Here's how the part is built. I have some questions about the finished solid (model axes, mm). A direction names the side the tool comes from. Round coordinates to 2 decimals unless told otherwise and drop trailing zeros. Order: outer loops, then holes, each group sorted by start corner. A loop starts at its lowest first (then second) coordinate and runs counter-clockwise, first axis right, second up.
Autodesk Inventor part; units mm, degrees
ref_plane "YZ Plane" through (0, 0, 0) normal (1, 0, 0) x (0, 1, 0)
ref_plane "XZ Plane" through (0, 0, 0) normal (0, 1, 0) x (-1, 0, 0)
ref_plane "XY Plane" through (0, 0, 0) normal (0, 0, 1) x (1, 0, 0)
ref_plane "Arbeitsebene1" through (796.2209, 70.6141, -996.2958) normal (0, 0, -1) x (-1, 0, 0)
sketch "Skizze1" plane through (796.2209, 70.6141, -996.2958) normal (0, 0, -1) x (-1, 0, 0)
  line L0 (-3.9996, -76.75) -> (4.0004, -76.75) construction
  line L1 (-3.9996, 76.75) -> (-3.9996, -76.75) construction
  line L2 (4.0004, 76.75) -> (-3.9996, 76.75) construction
  line L3 (4.0004, 84.25) -> (4.0004, 76.75) construction
  line L4 (-37.8996, 84.25) -> (4.0004, 84.25) construction
  line L5 (-37.8996, 1.75) -> (-37.8996, 84.25) construction
  line L6 (-133.3996, 1.75) -> (-37.8996, 1.75) construction
  line L7 (-133.3996, -84.25) -> (-133.3996, 1.75) construction
  line L8 (4.0004, -84.25) -> (-133.3996, -84.25) construction
  line L9 (4.0004, -76.75) -> (4.0004, -84.25) construction
  line L10 (150.8004, -76.75) -> (142.8004, -76.75) construction
  line L11 (142.8004, -76.75) -> (142.8004, -84.25) construction
  line L12 (142.8004, -84.25) -> (280.2004, -84.25) construction
  line L13 (280.2004, -84.25) -> (280.2004, 1.75) construction
  line L14 (280.2004, 1.75) -> (184.7004, 1.75) construction
  line L15 (184.7004, 1.75) -> (184.7004, 84.25) construction
  line L16 (184.7004, 84.25) -> (142.8004, 84.25) construction
  line L17 (142.8004, 84.25) -> (142.8004, 76.75) construction
  line L18 (142.8004, 76.75) -> (150.8004, 76.75) construction
  line L19 (150.8004, 76.75) -> (150.8004, -76.75) construction
  line L20 (-5.9996, 76.75) -> (-5.9996, -76.75) construction
  line L21 (152.8004, 76.75) -> (152.8004, -76.75) construction
  line L22 (-5.9996, 76.75) -> (152.8004, 76.75) construction
  line L23 (-5.9996, -76.75) -> (152.8004, -76.75) construction
  line L24 (73.4004, -76.75) -> (73.4004, 76.75) construction
  line L25 (-5.8996, -76.65) -> (152.7004, -76.65)
  line L26 (152.7004, -76.65) -> (152.7004, 76.65)
  line L27 (152.7004, 76.65) -> (-5.8996, 76.65)
  line L28 (-5.8996, 76.65) -> (-5.8996, -76.65)
  line L29 (-5.8996, -76.65) -> (152.7004, 76.65) construction
  line L30 (152.7004, -76.65) -> (-5.8996, 76.65) construction
  point P0 (796.2209, -70.6141)
  point P1 (73.4004, 0)
  dimension "d24" = 0.1
  dimension "d25" = 0.1
extrude "Extrusion1" add sketch "Skizze1" along normal blind 2
sketch "Skizze2" plane through (796.2209, 70.6141, -996.2958) normal (0, 0, 1) x (1, 0, 0)
  line L0 (-152.8004, -76.75) -> (-142.8004, -76.75) construction
  line L1 (-142.8004, -66.75) -> (-152.8004, -66.75) construction
  line L2 (-142.8004, -76.75) -> (-142.8004, -66.75) construction
  line L3 (-152.8004, -66.75) -> (-152.8004, -76.75) construction
  line L4 (-4.0004, -66.75) -> (5.9996, -66.75) construction
  line L5 (-4.0004, -76.75) -> (-4.0004, -66.75) construction
  line L6 (5.9996, -66.75) -> (5.9996, -76.75) construction
  line L7 (5.9996, -76.75) -> (-4.0004, -76.75) construction
  line L8 (-152.8004, 66.75) -> (-142.8004, 66.75) construction
  line L9 (-142.8004, 66.75) -> (-142.8004, 76.75) construction
  line L10 (-142.8004, 76.75) -> (-152.8004, 76.75) construction
  line L11 (-152.8004, 76.75) -> (-152.8004, 66.75) construction
  line L12 (-4.0004, 66.75) -> (-4.0004, 76.75) construction
  line L13 (5.9996, 66.75) -> (-4.0004, 66.75) construction
  line L14 (-4.0004, 76.75) -> (5.9996, 76.75) construction
  line L15 (5.9996, 76.75) -> (5.9996, 66.75) construction
  line L16 (-142.9004, -76.65) -> (-152.7004, -76.65)
  line L17 (-152.7004, -76.65) -> (-152.7004, -66.85)
  line L18 (-152.7004, -66.85) -> (-142.9004, -66.85)
  line L19 (-142.9004, -66.85) -> (-142.9004, -76.65)
  line L20 (5.8996, -76.65) -> (-152.7004, -76.65)
  line L21 (5.8996, -76.65) -> (5.8996, -66.85)
  line L22 (5.8996, -66.85) -> (-3.9004, -66.85)
  line L23 (-3.9004, -66.85) -> (-3.9004, -76.65)
  line L24 (-3.9004, -76.65) -> (5.8996, -76.65)
  line L25 (5.8996, 76.65) -> (5.8996, -76.65)
  line L26 (-3.9004, 66.85) -> (-3.9004, 76.65)
  line L27 (-3.9004, 76.65) -> (5.8996, 76.65)
  line L28 (5.8996, 76.65) -> (5.8996, 66.85)
  line L29 (5.8996, 66.85) -> (-3.9004, 66.85)
  line L30 (-142.9004, 76.65) -> (-142.9004, 66.85)
  line L31 (-142.9004, 66.85) -> (-152.7004, 66.85)
  line L32 (-152.7004, 66.85) -> (-152.7004, 76.65)
  line L33 (-152.7004, 76.65) -> (-142.9004, 76.65)
  line L34 (-152.7004, 76.65) -> (5.8996, 76.65)
  point P0 (-796.2209, -70.6141)
extrude "Extrusion2" add sketch "Skizze2" along normal blind 3.5
sketch "Skizze3" plane through (796.2209, 70.6141, -992.7958) normal (0, 0, 1) x (1, 0, 0)
  circle A0 centre (0.9996, 71.75) radius 1.75 construction
  circle A1 centre (0.9996, -71.75) radius 1.75 construction
  circle A2 centre (-147.8004, 71.75) radius 1.75 construction
  circle A3 centre (-147.8004, -71.75) radius 1.75 construction
  line L0 (-142.9004, 66.85) -> (-142.9004, 76.65)
  line L1 (-142.9004, 76.65) -> (-152.7004, 76.65)
  line L2 (-152.7004, 76.65) -> (-152.7004, 66.85)
  line L3 (-152.7004, 66.85) -> (-142.9004, 66.85)
  circle A4 centre (-147.8004, 71.75) radius 1.5
  circle A5 centre (1.0996, 71.75) radius 1.5
  circle A6 centre (1.0996, -71.75) radius 1.5
  circle A7 centre (-147.8004, -71.75) radius 1.5
  point P0 (-796.2209, -70.6141)
extrude "Extrusion3" cut sketch "Skizze3" against normal blind 15.5 contours A4 | A5 | A6 | A7
sketch "Skizze4" plane through (796.2209, 70.6141, -998.2958) normal (0, 0, -1) x (-1, 0, 0)
  circle A0 centre (147.8004, 71.75) radius 1.5 construction
  circle A1 centre (147.8004, -71.75) radius 1.5 construction
  circle A2 centre (-1.0996, -71.75) radius 1.5 construction
  circle A3 centre (147.8004, -71.75) radius 2.85
  circle A4 centre (-1.0996, -71.75) radius 2.85
  circle A5 centre (147.8004, 71.75) radius 2.85
  circle A6 centre (-1.0996, 71.75) radius 2.85
  circle A7 centre (-1.0996, 71.75) radius 1.5 construction
  point P0 (796.2209, -70.6141)
  dimension "d27" = 5.7
  dimension "d28" = 5.7
  dimension "d29" = 5.7
  dimension "d30" = 5.7
extrude "Extrusion4" cut sketch "Skizze4" against normal blind 3.1
equation "\"d28\" = d27"
equation "\"d29\" = d27"
equation "\"d30\" = d27"
properties part number "Backplate-housing"
1. If we section it at A-A, the plane y = 130.5: Write out the boundary of the cut face in (x, z), and give its area (3 significant figures).
Evaluation:
outline: (643.52, -998.3) - (802.12, -998.3) - (802.12, -996.3) - (643.52, -996.3) - close
area: 317 mm2
2. If we mould it in two halves opening along Y, with no side actions, what happens to faces 1 (the flat face through (647, -2, -995.196)), 2 (the flat face through (792.32, -1, -995))? For each: released by +Y, released by -Y, zero draft, split by the parting line, or undercut.
Evaluation:
face 1: undercut
face 2: zero draft
3. On a 3-axis mill with a long thin cutter (end or side, diameter ignored), from which of +Z, -Z, +X, -X, +Y, -Y can I reach the whole of each face in a straight line? I mean faces 3 (the cylindrical face through (794.69, 141.27, -996.77)), 4 (the flat face through (648, 137.464, -995)), 5 (the flat face through (653.32, -1, -995)). Say none if no direction works.
Evaluation:
face 3: -Z
face 4: +Z, +X, -X
face 5: +Z, +Y, -Y
4. I need wall thicknesses on probe 1 along Z at (x, y) = (749, 105.5). Which ranges of the line are inside material? Lowest first, please.
Evaluation:
probe 1: z = -998.3 to -996.3
5. If we section it at B-B, the plane x = 782: Write out the boundary of the cut face in (y, z).
Evaluation:
outline: (-6.04, -998.3) - (147.26, -998.3) - (147.26, -996.3) - (-6.04, -996.3) - close
6. I'm going to push flat-ended pins straight in: P1, Ø6, axis at x = 745, y = 19.5, coming from the +Z side; P2, Ø5, axis at x = 648.42, y = -1.14, coming from the +Z side. Where does each tip first touch, or does it pass through?
Evaluation:
P1: stops at z = -996.3
P2: stops at z = -992.8
